Source: CAD feature listing. Evaluate the final solid. Frame: model axes, mm. A direction names the side the tool comes from. Round coordinates to 2 decimals unless told otherwise and drop trailing zeros. Order: outer loops, then holes, each group sorted by start corner. A loop starts at its lowest first (then second) coordinate and runs counter-clockwise, first axis right, second up. Notation, with made-up numbers: (42, -4) - (70, -4) arc R22 cw to (70, 3) - close; hole circle Ø10 at (89.25, -14). An arc over 180 degrees is marked (long way). Put each result on its own line as item: value. Start each with the question number.
1) Access query for faces 1 (the face through (-37, 21.258, 1)), 2 (the face through (-33.868, 20.555, 4.493)), 3 (the face through (-32.831, 25, 1)). Directions: +Z, -Z, +X, -X, +Y, -Y. A direction counts if a zero-diameter tool reaches every point of the face in a straight line with its end or side. Return the directions, or none.
2) Section B-B on y = 16. Output: boundary loops of the cut face in (x, z), then the cut area to 3 significant figures.
3) Mould query, pull axis X, two halves, no side actions, for faces 4 (the face through (-30.825, 15.46, 4.493)), 5 (the face through (-31.1, 23.8, 5)), 6 (the face through (-30.893, 24.053, 4.493)). Classes: +X half, -X half, draft (parallel to the pull), parting line (faces both ways), or undercut.
4) Section A-A on z = 0.6. Output: boundary loops of the cut face in (x, y).
5) Section C-C on z = 4.4. State how many separate pieces and enclosed holes the cut face has, then the cut area to 3 significant figures.
6) Contact query for flat-ended pins moving along their axis: P1, Ø0.6, axis at x = -35.5, z = 1, coming from the -Y side; P2, Ø1, axis at y = 16, z = 1.5, coming from the +X side; P3, Ø1, axis at x = -27, z = 0.5, coming from the +Y side. Output: stop coordinate, or through.
7) Section D-D on y = 26.75. Output: boundary loops of the cut face in (x, z), then the cut area to 3 significant figures.
8) Line query: probe 1 along X at (y, z) = (14.5, 4.15); probe 2 along X at (y, z) = (23, 4.4); probe 3 along Z at (x, y) = (-32.5, 12.25). Output: solid intervals per line, ascending. Write a range as [from, to].
```python
from build123d import *

# Parameters (mm, degrees)
F0_R     = 9
F1_DEPTH = 4
F3_W     = 3
F3_H     = 3
F4_DEPTH = 2
F2_R     = 9
F2_R_2   = 8
F5_DEPTH = 1
F7_DEPTH = 1


# Not quite as in the source:
# - a feature names something its author has since deleted; it is built from what else it names


with BuildPart() as f1:
    # F0 (on Top) → F1 (new body)
    with BuildSketch(Plane.XY):
        with Locations((-31.3306450844, 19.7580661625)):
            Circle(F0_R)
    extrude(amount=F1_DEPTH)

    # F3 (on face) → F4 (cut)
    with BuildSketch(Plane(origin=(0, 0, 0), x_dir=(1, 0, 0), z_dir=(0, 0, -1))):
        with BuildLine():
            ThreePointArc((-32.8306450844, -28.6321858371), (-32.0832814269, -28.7265408676), (-31.3306450844, -28.7580661625))
            ThreePointArc((-31.3306450844, -28.7580661625), (-30.5780087419, -28.7265408676), (-29.8306450844, -28.6321858371))
            Line((-29.8306450844, -28.6321858371), (-29.8306450844, -21.2580661625))
            Line((-29.8306450844, -21.2580661625), (-32.8306450844, -21.2580661625))
            Line((-32.8306450844, -21.2580661625), (-32.8306450844, -28.6321858371))
        make_face()
        with BuildLine():
            ThreePointArc((-40.204764759, -18.2580661625), (-40.2991197895, -19.0054298199), (-40.3306450844, -19.7580661625))
            ThreePointArc((-40.3306450844, -19.7580661625), (-40.2991197895, -20.510702505), (-40.204764759, -21.2580661625))
            Line((-40.204764759, -21.2580661625), (-32.8306450844, -21.2580661625))
            Line((-32.8306450844, -21.2580661625), (-32.8306450844, -18.2580661625))
            Line((-32.8306450844, -18.2580661625), (-40.204764759, -18.2580661625))
        make_face()
        with Locations((-31.3306450844, -19.7580661625)):
            Rectangle(F3_W, F3_H)
        with BuildLine():
            Line((-29.8306450844, -18.2580661625), (-29.8306450844, -21.2580661625))
            Line((-29.8306450844, -21.2580661625), (-22.4565254097, -21.2580661625))
            ThreePointArc((-22.4565254097, -21.2580661625), (-22.3621703793, -20.510702505), (-22.3306450844, -19.7580661625))
            ThreePointArc((-22.3306450844, -19.7580661625), (-22.3621703793, -19.0054298199), (-22.4565254097, -18.2580661625))
            Line((-22.4565254097, -18.2580661625), (-29.8306450844, -18.2580661625))
        make_face()
        with BuildLine():
            Line((-32.8306450844, -10.8839464878), (-32.8306450844, -18.2580661625))
            Line((-32.8306450844, -18.2580661625), (-29.8306450844, -18.2580661625))
            Line((-29.8306450844, -18.2580661625), (-29.8306450844, -10.8839464878))
            ThreePointArc((-29.8306450844, -10.8839464878), (-30.5780087419, -10.7895914574), (-31.3306450844, -10.7580661625))
            ThreePointArc((-31.3306450844, -10.7580661625), (-32.0832814269, -10.7895914574), (-32.8306450844, -10.8839464878))
        make_face()
    extrude(amount=-F4_DEPTH, mode=Mode.SUBTRACT)

    # F2 (on face) → F5 (join)
    with BuildSketch(Plane.XY.offset(4)):
        with Locations((-31.3306450844, 19.7580661625)):
            Circle(F2_R)
        with Locations((-31.3306450844, 19.7580661625)):
            Circle(F2_R_2, mode=Mode.SUBTRACT)
    extrude(amount=F5_DEPTH)

    # F6 (on face) → F7 (join)
    with BuildSketch(Plane.XY.offset(4)):
        Polygon((-31.9784342899, 25.4181322135), (-31.7774611038, 25.2590085979), (-31.1892692607, 24.7560993929), (-30.7208457687, 24.5338144768), (-30.4025390075, 24.6978790801), (-30.392716562, 24.8693254), (-30.4025390075, 25.1047664399), (-30.8471683696, 25.5198689359), (-31.6626039755, 25.7905517194), (-31.8783703596, 25.8094227206), (-32.0071634544, 25.7774551255), (-32.085100094, 25.7093528374), (-32.0432445706, 25.5871378045), align=None)
        Polygon((-32.0727952488, 23.82088353), (-34.1039519464, 23.641281604), (-34.4009291186, 23.5190665711), (-34.2549080498, 23.3492275605), (-33.6609834704, 23.1039640751), (-32.9981350893, 23.1326575217), (-28.9325058746, 23.7331363511), (-28.1966558885, 23.8783299532), (-27.8397737053, 24.0251903945), (-27.7799460833, 24.1039485477), (-27.774171676, 24.2417604333), (-27.925973105, 24.373024022), (-28.2204678774, 24.520658353), (-28.8430918564, 24.514110056), (-29.7462805942, 24.2778355965), align=None)
        Polygon((-34.382885584, 20.0842467066), (-33.3393966077, 21.0391074603), (-33.2631029954, 20.8914731293), (-33.073613141, 20.7339568229), (-32.8504769463, 20.4394620505), (-32.5781154176, 20.1235960182), (-32.2860792331, 19.9595314149), (-32.1999334103, 19.9800692553), (-32.1088704119, 20.0842467066), (-32.0826236472, 20.5436395019), (-32.3664685075, 20.8693279796), (-33.0604867821, 21.2294247813), (-33.1507282669, 21.2310916205), (-33.1753379574, 21.255677499), (-33.1457872792, 21.3246132068), (-33.0227447798, 21.5075488113), (-32.8135564575, 21.7938284475), (-32.5256159351, 22.1711889411), (-32.4854153449, 22.3016191102), (-32.5649890587, 22.4894957023), (-33.0170120434, 22.7807163262), (-33.3525229666, 22.866856196), (-33.4591649588, 22.8061356243), (-33.4673741419, 22.6765388749), (-33.689688823, 21.578925248), (-34.4845925415, 20.4550589033), (-34.7323443797, 20.1843165898), (-34.9046181661, 20.0087627019), (-34.9333294717, 19.8783325328), (-34.8291579734, 19.8807732617), (-34.6355486449, 19.9373862652), align=None)
        Polygon((-35.6429326931, 17.8857095862), (-31.560897018, 18.5354375615), (-31.5518663213, 16.6232038893), (-31.5215238944, 15.2286190431), (-31.4698399726, 14.3401836183), (-31.3968205087, 13.9447772089), (-31.3992731436, 13.8832511968), (-31.3443150733, 13.8561793466), (-31.1671300641, 13.7905517194), (-31.0005771079, 14.0834147752), (-30.8619318027, 14.7323117121), (-30.786507328, 16.2089407659), (-30.8094263673, 16.546904324), (-30.8012707611, 17.064559103), (-30.775851463, 17.7519993157), (-30.7470984864, 18.5977892544), (-30.2294853783, 18.5887585576), (-29.2737316751, 18.6067961392), (-27.8980535481, 18.6330488569), (-26.120369519, 18.6502887368), (-25.8890360471, 18.6707849062), (-25.726578753, 18.7749742635), (-25.7462831738, 18.9521771317), (-25.8939175048, 19.1818616234), (-26.8102623665, 19.6675071364), (-27.4952737563, 19.6675071364), (-28.9505434561, 19.4410967932), (-30.7340018925, 19.1687352645), (-30.7569209318, 19.1884337323), (-30.7208457687, 19.2343670588), (-30.6872113344, 19.6199188766), (-30.6060124524, 20.0350154196), (-30.6355393186, 20.2318810376), (-30.7602546103, 20.4156500617), (-30.9349750786, 20.502623351), (-31.0391525299, 20.5928707888), (-30.5207060022, 20.9111775501), (-29.8480173166, 21.5214788248), (-29.7602701377, 21.3886079269), (-29.5789418424, 21.255677499), (-29.0776994767, 20.8209301122), (-28.5387151086, 20.3664187747), (-28.4132259273, 20.2647415822), (-28.2466610651, 20.2515854584), (-28.17201048, 20.2655750018), (-28.0924784372, 20.3893973439), (-28.0924784372, 20.5501877988), (-28.1318277488, 20.8225374215), (-28.5707422337, 21.2827636364), (-29.618291154, 21.7249522697), (-29.6593073048, 21.7101888366), (-29.6707965895, 21.7249522697), (-29.2992105032, 22.2466729458), (-28.8668443153, 22.8275068844), (-28.8373174491, 22.9825229319), (-28.9062531568, 23.1457541156), (-29.3689201006, 23.4369747395), (-29.6937751587, 23.5296629062), (-29.8111087339, 23.461620148), (-29.8086084751, 23.3262489912), (-29.8455765878, 22.8619152083), (-30.0095816611, 22.3566248045), (-30.3074101119, 21.8037104229), (-30.7470984864, 21.1933496182), (-30.9267599424, 21.0588118811), (-31.2163375391, 20.6847255359), (-31.342677999, 20.7191933898), (-31.419793125, 20.7602095406), (-31.620772264, 20.7790805418), (-31.8135600789, 20.7077041052), (-31.9062541986, 20.5534619473), (-31.8398127967, 20.4419027794), (-31.6757303344, 19.9152411156), (-31.5871497358, 19.2474934177), (-31.6084674188, 19.1621869676), (-31.5740233769, 19.067010448), (-36.6470354491, 18.5354375615), (-36.8504809149, 18.4361653799), (-36.7356315255, 18.2302750181), (-36.2385062527, 17.9037709798), align=None)
    extrude(amount=F7_DEPTH)


solid = f1.part
```
Answer sheet:
1. face 1: -Z, +X, -X
1. face 2: +Z
1. face 3: -Z, +Y, -Y
2. outline: (-39.51, 0) - (-32.83, 0) - (-32.83, 2) - (-29.83, 2) - (-29.83, 0) - (-23.15, 0) - (-23.15, 5) - (-24.27, 5) - (-24.27, 4) - (-30.8, 4) - (-30.8, 5) - (-31.54, 5) - (-31.54, 4) - (-38.39, 4) - (-38.39, 5) - (-39.51, 5) - close
2. area: 62.4 mm^2
3. face 4: undercut
3. face 5: draft
3. face 6: undercut
4. outline: (-40.2, 18.26) arc R9 ccw to (-32.83, 10.88) - (-32.83, 18.26) - close; (-40.2, 21.26) - (-32.83, 21.26) - (-32.83, 28.63) arc R9 ccw to start; (-29.83, 10.88) arc R9 ccw to (-22.46, 18.26) - (-29.83, 18.26) - close; (-29.83, 21.26) - (-22.46, 21.26) arc R9 ccw to (-29.83, 28.63) - close
5. separate pieces: 5
5. enclosed holes: 1
5. area: 77.1 mm^2
6. P1: y = 11.63
6. P2: x = -22.94
6. P3: y = 27.9
7. outline: (-37, 0) - (-32.83, 0) - (-32.83, 2) - (-29.83, 2) - (-29.83, 0) - (-25.66, 0) - (-25.66, 5) - (-27.44, 5) - (-27.44, 4) - (-35.22, 4) - (-35.22, 5) - (-37, 5) - close
7. area: 42.9 mm^2
8. probe 1: [-38.63, -37.36], [-31.48, -30.91], [-25.3, -24.03]
8. probe 2: [-39.73, -38.64], [-29.83, -28.84], [-24.02, -22.93]
8. probe 3: [2, 4]
